Verification items for the finished model (mm, model axes). A direction names the side the tool comes from. Round coordinates to 2 decimals unless told otherwise and drop trailing zeros. Write each loop counter-clockwise with the first axis right and the second up, starting at its lowest first coordinate (ties: lowest second). Pieces come first, ordered by that corner, then holes. Notation, with made-up numbers: (84.5, -30) - (135.5, -30) arc R29 cw to (135.5, 1) - close; hole circle Ø5 at (-10.75, 57.5). An arc over 180 degrees is marked (long way). Answer as a JSON object with one key per item and string values.
```python
from build123d import *

# Parameters (mm, degrees)
SKETCH1_W           = 50
SKETCH1_H           = 20
BOSS_EXTRUDE1_DEPTH = 20
SKETCH2_R           = 2.75
SKETCH2_W           = 7
SKETCH2_H           = 5
CUT_EXTRUDE1_DEPTH  = 21
SKETCH3_R           = 2.25
CUT_EXTRUDE2_DEPTH  = 21
SKETCH5_W           = 8
SKETCH5_H           = 6
BOSS_EXTRUDE3_DEPTH = 3
SKETCH6_R           = 4.5
CUT_EXTRUDE3_DEPTH  = 5
SKETCH7_W           = 10
SKETCH7_H           = 20
CUT_EXTRUDE4_DEPTH  = 24


with BuildPart() as part:
    # Sketch1 → Boss-Extrude1 (new body)
    with BuildSketch(Plane.XY):
        with Locations((25, 10)):
            Rectangle(SKETCH1_W, SKETCH1_H)
    extrude(amount=BOSS_EXTRUDE1_DEPTH)

    # Sketch2 → Cut-Extrude1 (cut, through all)
    with BuildSketch(Plane.XY.offset(20)):
        with Locations((25, 10)):
            Circle(SKETCH2_R)
        with Locations((45, 10)):
            Circle(SKETCH2_R)
        with Locations((15, 10)):
            Rectangle(SKETCH2_W, SKETCH2_H)
    extrude(amount=-CUT_EXTRUDE1_DEPTH, mode=Mode.SUBTRACT)

    # Sketch3 → Cut-Extrude2 (cut, through all)
    with BuildSketch(Plane(origin=(0, 20, 0), x_dir=(1, 0, 0), z_dir=(0, 1, 0))):
        with Locations((15, -11.5)):
            Circle(SKETCH3_R)
    extrude(amount=-CUT_EXTRUDE2_DEPTH, mode=Mode.SUBTRACT)

    # Sketch5 → Boss-Extrude3 (add)
    with BuildSketch(Plane(origin=(0, 0, 0), x_dir=(-1, 0, 0), z_dir=(0, 0, -1))):
        with Locations((-35, 10)):
            Rectangle(SKETCH5_W, SKETCH5_H)
    extrude(amount=BOSS_EXTRUDE3_DEPTH)

    # Sketch6 → Cut-Extrude3 (cut)
    with BuildSketch(Plane.XY.offset(20)):
        with Locations((25, 10)):
            Circle(SKETCH6_R)
        with Locations((45, 10)):
            Circle(SKETCH6_R)
    extrude(amount=-CUT_EXTRUDE3_DEPTH, mode=Mode.SUBTRACT)

    # Sketch7 → Cut-Extrude4 (cut, through all)
    with BuildSketch(Plane.XY.offset(20)):
        with Locations((5, 10)):
            Rectangle(SKETCH7_W, SKETCH7_H)
    extrude(amount=-CUT_EXTRUDE4_DEPTH, mode=Mode.SUBTRACT)


solid = part.part
```
Q1. Set-up check for faces 1 (the cylindrical face through (49.292, 11.352, 17.535)), 2 (the flat face through (18.5, 10, 10)), 3 (the flat face through (35, 7, -1)), 4 (the flat face through (35, 13, -1)): record each of +Z, -Z, +X, -X, +Y, -Y from which the full face is reachable in a straight line by a thin tool's end or side.
Geometry check:
{"face 1": "+Z", "face 2": "+Z, -Z", "face 3": "-Z, +X, -X, -Y", "face 4": "-Z, +X, -X, +Y"}
Q2. Material ranges on line 1 along Y through (x, z) = (18, 5.75); line 2 along X through (y, z) = (9, 15.75); line 3 along X through (y, z) = (10.5, 1.5), recorded low to high. Write a range as [from, to].
Geometry check:
{"line 1": "y = [0, 7.5], [12.5, 20]", "line 2": "x = [10, 11.5], [18.5, 20.61], [29.39, 40.61], [49.39, 50]", "line 3": "x = [10, 11.5], [18.5, 22.3], [27.7, 42.3], [47.7, 50]"}
Q3. Release check for a two-part mould opening along Z. For faces 5 (the flat face through (30, 10, 20)), 6 (the flat face through (15, 12.5, 8)), 7 (the cylindrical face through (16.21, 16.303, 9.603)), 8 (the cylindrical face through (16.21, 3.803, 9.603)) record: released by +Z, released by -Z, zero draft, split by the parting line, or undercut.
Geometry check:
{"face 5": "released by +Z", "face 6": "zero draft", "face 7": "undercut", "face 8": "undercut"}
Q4. Section check D-D, the plane x = 45. Record the cut outline in (y, z).
Geometry check:
{"outline": "(0, 0) - (7.25, 0) - (7.25, 15) - (5.5, 15) - (5.5, 20) - (0, 20) - close; (12.75, 0) - (20, 0) - (20, 20) - (14.5, 20) - (14.5, 15) - (12.75, 15) - close"}
Q5. Section check C-C, the plane z = 10.5. Record the cut outline in (x, y), then the cut area to 3 significant figures.
Geometry check:
{"outline": "(10, 0) - (12.98, 0) - (12.98, 7.5) - (11.5, 7.5) - (11.5, 12.5) - (12.98, 12.5) - (12.98, 20) - (10, 20) - close; (17.02, 0) - (50, 0) - (50, 20) - (17.02, 20) - (17.02, 12.5) - (18.5, 12.5) - (18.5, 7.5) - (17.02, 7.5) - close; hole circle Ø5.5 at (25, 10); hole circle Ø5.5 at (45, 10)", "area": "657 mm2"}
Q6. Gauge pin test, flat ends, axial feed: P1, Ø2.5, axis at x = 25.5, y = 9, coming from the +Z side; P2, Ø2.5, axis at x = 47, y = 11, coming from the +Z side; P3, Ø0.9, axis at x = 35, z = -1.5, coming from the +Y side; P4, Ø1.5, axis at y = 11, z = -2, coming from the +X side. Record the tip position at first contact, or that the pin passes through.
Geometry check:
{"P1": "passes through", "P2": "stops at z = 15", "P3": "stops at y = 13", "P4": "stops at x = 39"}
Q7. Section check A-A, the plane x = 15. Record the cut outline in (y, z).
Geometry check:
{"outline": "(0, 0) - (7.5, 0) - (7.5, 9.25) - (0, 9.25) - close; (0, 13.75) - (7.5, 13.75) - (7.5, 20) - (0, 20) - close; (12.5, 0) - (20, 0) - (20, 9.25) - (12.5, 9.25) - close; (12.5, 13.75) - (20, 13.75) - (20, 20) - (12.5, 20) - close"}
Q8. Section check B-B, the plane z = 18. Record the cut outline in (x, y).
Geometry check:
{"outline": "(10, 0) - (50, 0) - (50, 20) - (10, 20) - close; hole (11.5, 7.5) - (18.5, 7.5) - (18.5, 12.5) - (11.5, 12.5) - close; hole circle Ø9 at (25, 10); hole circle Ø9 at (45, 10)"}
